from build123d import *

# Parameters (mm, degrees)
SKETCH1_R               = 6
BOSS_EXTRUDE1_DEPTH     = 17
SKETCH2_OUTSIDE_W       = 18.804
SKETCH2_OUTSIDE_H       = 18.804
SKETCH2_OUTSIDE_W_2     = 8.9
SKETCH2_OUTSIDE_H_2     = 8.9
CUT_EXTRUDE1_DEPTH      = 11.5
SKETCH3_R               = 5
BOSS_EXTRUDE2_DEPTH     = 3.5
CUT_EXTRUDE2_DEPTH      = 20
CUT_EXTRUDE2_DEPTH_BACK = 20
SKETCH5_W               = 1.5
SKETCH5_H               = 3.5
FILLET2_R               = 1
CUT_EXTRUDE3_DEPTH      = 7
CUT_EXTRUDE4_DEPTH      = 8
SKETCH8_R               = 1
CUT_EXTRUDE5_DEPTH      = 18.233688027
CHAMFER1_START          = -6
CHAMFER1_2_OUTLINE_W    = 10
CHAMFER1_2_OUTLINE_H    = 4
CHAMFER1_2_DEPTH        = 1.403805922


with BuildPart() as part:
    # Sketch1 → Boss-Extrude1 (new body)
    with BuildSketch(Plane(origin=(0, 0, 0), x_dir=(1, 0, 0), z_dir=(0, 1, 0))):
        with Locations(Location((0, 0, 0), (0, 0, 270))):
            Circle(SKETCH1_R)
    extrude(amount=BOSS_EXTRUDE1_DEPTH)

    # Sketch2 outside → Cut-Extrude1 (cut)
    with BuildSketch(Plane(origin=(0, 17, 0), x_dir=(1, 0, 0), z_dir=(0, 1, 0))):
        Rectangle(SKETCH2_OUTSIDE_W, SKETCH2_OUTSIDE_H)
        Rectangle(SKETCH2_OUTSIDE_W_2, SKETCH2_OUTSIDE_H_2, mode=Mode.SUBTRACT)
    extrude(amount=-CUT_EXTRUDE1_DEPTH, mode=Mode.SUBTRACT)

    # Sketch3 → Boss-Extrude2 (add)
    with BuildSketch(Plane.XZ):
        with Locations(Location((0, 0, 0), (0, 0, 270))):
            Circle(SKETCH3_R)
    extrude(amount=BOSS_EXTRUDE2_DEPTH)

    # Sketch4 → Cut-Revolve2 (revolve, cut)
    with BuildSketch(Plane(origin=(0, -7.347807266, 1), x_dir=(0, 0, -1), z_dir=(1, 0, 0))):
        with BuildLine():
            Line((0, 5.75), (0, -5.75))
            ThreePointArc((0, -5.75), (-5.75, 0), (0, 5.75))
        make_face()
    revolve(axis=Axis((0, -1.597807266, 1), (0, -1, 0)), mode=Mode.SUBTRACT)

    # Sketch5 → Cut-Extrude2 (cut, two sides: drawn at the far end of the back side and taken through both)
    with BuildSketch(Plane(origin=(0, 0, 0), x_dir=(0, 0, -1), z_dir=(1, 0, 0)).offset(-CUT_EXTRUDE2_DEPTH_BACK)):
        with Locations((4.25, -1.75)):
            Rectangle(SKETCH5_W, SKETCH5_H)
    extrude(amount=CUT_EXTRUDE2_DEPTH + CUT_EXTRUDE2_DEPTH_BACK, mode=Mode.SUBTRACT)

    # Fillet2
    fillet2_edges = [part.edges().sort_by_distance(p)[0] for p in [
        (0, 0, -3.5),
    ]]
    fillet(fillet2_edges, radius=FILLET2_R)

    # Sketch6 → Cut-Extrude3 (cut)
    with BuildSketch(Plane.XZ.offset(3.5)):
        with BuildLine():
            Line((2.1, -2.1), (-2.1, -2.1))
            ThreePointArc((-2.1, -2.1), (-2.807106781, -1.807106781), (-3.1, -1.1))
            Line((-3.1, -1.1), (-3.1, 3.1))
            ThreePointArc((-3.1, 3.1), (-2.807106781, 3.807106781), (-2.1, 4.1))
            Line((-2.1, 4.1), (2.1, 4.1))
            ThreePointArc((2.1, 4.1), (2.807106781, 3.807106781), (3.1, 3.1))
            Line((3.1, 3.1), (3.1, -1.1))
            ThreePointArc((3.1, -1.1), (2.807106781, -1.807106781), (2.1, -2.1))
        make_face()
    extrude(amount=-CUT_EXTRUDE3_DEPTH, mode=Mode.SUBTRACT)

    # Sketch7 → Cut-Extrude4 (cut)
    with BuildSketch(Plane.XZ.offset(-3.5)):
        with BuildLine():
            Line((2.1, -1.1), (-2.1, -1.1))
            ThreePointArc((-2.1, -1.1), (-2.807106781, -0.807106781), (-3.1, -0.1))
            Line((-3.1, -0.1), (-3.1, 2.1))
            ThreePointArc((-3.1, 2.1), (-2.807106781, 2.807106781), (-2.1, 3.1))
            Line((-2.1, 3.1), (2.1, 3.1))
            ThreePointArc((2.1, 3.1), (2.807106781, 2.807106781), (3.1, 2.1))
            Line((3.1, 2.1), (3.1, -0.1))
            ThreePointArc((3.1, -0.1), (2.807106781, -0.807106781), (2.1, -1.1))
        make_face()
    extrude(amount=-CUT_EXTRUDE4_DEPTH, mode=Mode.SUBTRACT)

    # Sketch8 → Cut-Extrude5 (cut, through all)
    with BuildSketch(Plane.XZ.offset(-11.5)):
        with Locations(Location((0, 1.043592984, 0), (0, 0, 270))):
            Circle(SKETCH8_R)
    extrude(amount=-CUT_EXTRUDE5_DEPTH, mode=Mode.SUBTRACT)

    # Chamfer1: read off the stored shape, not the designer's step
    # Chamfer1 outline → Chamfer1 (revolve, cut)
    with BuildSketch(Plane.XY):
        Polygon((5, -3), (4.5, -3.5), (5, -3.5), align=None)
    revolve(axis=Axis((0, 0, 0), (0, 1, 0)), mode=Mode.SUBTRACT)

    # Chamfer1 2 outline → Chamfer1 2 (cut)
    with BuildSketch(Plane(origin=(0, 0, 0), x_dir=(1, 0, 0), z_dir=(0, 0.707106781186544, 0.707106781186551)).offset(CHAMFER1_START)):
        Rectangle(CHAMFER1_2_OUTLINE_W, CHAMFER1_2_OUTLINE_H)
    extrude(amount=CHAMFER1_2_DEPTH, mode=Mode.SUBTRACT)


solid = part.part
Design review of the part built by this model. Coordinates are the model's own, in mm. A direction names the side the tool comes from. Round coordinates to 2 decimals unless told otherwise and drop trailing zeros. Write each loop counter-clockwise with the first axis right and the second up, starting at its lowest first coordinate (ties: lowest second). Pieces come first, ordered by that corner, then holes. Notation, with made-up numbers: (11.5, 81.25) - (29.5, 81.25) arc R18 cw to (29.5, 95.25) - close; hole circle Ø5 at (-6.5, 87). An arc over 180 degrees is marked (long way). Return JSON: item names as keys, results as strings. Group by question number.
Item 1: For probe 1 along X at (y, z) = (9.25, -1.25); probe 2 along Y at (x, z) = (-1, 4); probe 3 along X at (y, z) = (9, 3), list the stretches that pass through material, from the lowest coordinate up. Write a range as [from, to].
Item 2: We need section D-D on y = 1.25. Write out the cut boundary in (x, z).
Item 3: Machinability: for faces 1 (the face through (0, 5.5, 5)), 2 (the face through (0, -2, -3.5)), 3 (the face through (-5, 5.5, 0)), 4 (the face through (4.45, 11, 0)), 5 (the face through (2.799, 0.109, 3.815)), which of the approach directions +Z, -Z, +X, -X, +Y, -Y give a long, thin tool a straight path to every point of the face, cutting with its end or side? Answer none if there is none.
Item 4: We need section A-A on y = 15.75. Write out the cut boundary in (x, z), and give its area (3 significant figures).
Item 5: We need section C-C on y = 7.25. Write out the cut boundary in (x, z).
Item 6: We need section B-B on x = 0. Write out the cut boundary in (y, z).
Item 7: Insertion check: P1, Ø0.6, axis at x = 0.5, y = -2, coming from the -Z side; P2, Ø1.5, axis at y = 1.5, z = -4, coming from the -X side; P3, Ø0.6, axis at x = -1, z = -1.5, coming from the -Y side; P4, Ø1.8, axis at x = 0, z = 1.04, coming from the -Y side. Each pin has a flat end and moves straight along its axis. Give the tip position at first contact, or say it passes through.
Model answer:
{
 "1": {"probe 1": "x = [-4.45, 4.45]", "probe 2": "y = [3.5, 17]", "probe 3": "x = [-4.45, -2.54], [2.54, 4.45]"},
 "2": {"outline": "circle Ø12 at (0, 0); hole (-3.1, -1.1) arc R1 ccw to (-2.1, -2.1) - (2.1, -2.1) arc R1 ccw to (3.1, -1.1) - (3.1, 3.1) arc R1 ccw to (2.1, 4.1) - (-2.1, 4.1) arc R1 ccw to (-3.1, 3.1) - close"},
 "3": {"face 1": "+Z, +X, -X, +Y", "face 2": "-Z, +X, -X, -Y", "face 3": "+Z, -Z, -X, +Y", "face 4": "+Z, -Z, +X, +Y", "face 5": "-Y"},
 "4": {"outline": "(-4.45, -4.02) arc R6 ccw to (-4.02, -4.45) - (4.02, -4.45) arc R6 ccw to (4.45, -4.02) - (4.45, 4.02) arc R6 ccw to (4.02, 4.45) - (-4.02, 4.45) arc R6 ccw to (-4.45, 4.02) - close; hole circle Ø2 at (0, 1.04)", "area": "75.7 mm²"},
 "5": {"outline": "(-4.45, -4.02) arc R6 ccw to (-4.02, -4.45) - (4.02, -4.45) arc R6 ccw to (4.45, -4.02) - (4.45, 4.02) arc R6 ccw to (4.02, 4.45) - (-4.02, 4.45) arc R6 ccw to (-4.45, 4.02) - close; hole (-3.1, -0.1) arc R1 ccw to (-2.1, -1.1) - (2.1, -1.1) arc R1 ccw to (3.1, -0.1) - (3.1, 2.1) arc R1 ccw to (2.1, 3.1) - (-2.1, 3.1) arc R1 ccw to (-3.1, 2.1) - close"},
 "6": {"outline": "(-3.36, -3.14) - (-3, -3.5) - (-1, -3.5) arc R1 cw to (0, -4.5) - (0, -6) - (5.5, -6) - (5.5, -4.45) - (17, -4.45) - (17, 0.04) - (11.5, 0.04) - (11.5, -1.1) - (3.5, -1.1) - (3.5, -2.1) - (-2.51, -2.1) arc R5.75 cw to start; (-3.11, 4.89) arc R5.75 cw to (-2.51, 4.1) - (3.5, 4.1) - (3.5, 3.1) - (11.5, 3.1) - (11.5, 2.04) - (17, 2.04) - (17, 4.45) - (5.5, 4.45) - (5.5, 6) - (0, 6) - (0, 5) - (-3, 5) - close"},
 "7": {"P1": "stops at z = -3.5", "P2": "stops at x = -5.04", "P3": "stops at y = 3.5", "P4": "passes through"}
}
